For this review, take the finished solid that the model builds, in its own axes (mm). A direction names the side the tool comes from. Round coordinates to 2 decimals unless told otherwise and drop trailing zeros. Write each loop counter-clockwise with the first axis right and the second up, starting at its lowest first coordinate (ties: lowest second). Pieces come first, ordered by that corner, then holes. Notation, with made-up numbers: M 2,42.5 L 42,42.5 A25 ccw 42,72.5 Z; hole C 59,-19 d7. An arc over 180 degrees is marked long. Use one line per item in the form item = value. Start each with the question number.
Item 1: For faces 5 (the cylindrical face through (-0.43, 36.18, 19.26)), 6 (the cylindrical face through (-0.16, -36.18, 22.38)), 7 (the flat face through (0, 39.933, 32)), list the 3-axis set-ups (+Z, -Z, +X, -X, +Y, -Y) from which the entire face can be reached by the end or side of a thin tool; tool diameter is ignored.
Item 2: For line 1 (X direction, y = 9, z = 13.5); line 2 (Y direction, x = 7.5, z = 16); line 3 (Y direction, x = 28, z = 10.5), list the stretches that pass through material, from the lowest coordinate up. Write a range as [from, to].
Item 3: Add section A-A (y = 0). State the section outline as (x, z) points.
Item 4: Draft analysis for pull direction X (two halves, no side actions). For faces 1 (the cylindrical face through (-0.15, -0.559, 33.453)), 2 (the flat face through (51.073, 0, 22)), 3 (the cylindrical face through (-22.66, -4.07, 22.92)), 4 (the flat face through (1, 32.313, 18)), state which applies: released by +X, released by -X, zero draft, split by the parting line, or undercut.
Item 5: Add section C-C (z = 8.5). State the section outline as (x, y) points, and give its area (4 significant figures).
Item 6: Add section B-B (z = 36). State the section outline as (x, y) points.
Item 7: Add section D-D (y = 17). State the section outline as (x, z) points.
Item 8: For P1, Ø4, axis at x = -30, z = 21, coming from the -Y side; P2, Ø10, axis at x = -11, z = 14.5, coming from the +Y side, all flat-tipped, find the tip position at first contact; note any pin that passes through.
from build123d import *

# Parameters (mm, degrees)
F0_W      = 102.14658
F0_H      = 79.865314
F1_DEPTH  = 45.212
F3_DEPTH  = 7.62
F5_DEPTH  = 7.62
F8_DEPTH  = 240.792
F9_R      = 10.614666
F9_R_2    = 10.738577
F10_DEPTH = 83.566


with BuildPart() as f1:
    # F0 (on Top) → F1 (new body)
    with BuildSketch(Plane.XY):
        Rectangle(F0_W, F0_H)
    extrude(amount=F1_DEPTH)

    # F2 (on face) → F3 (cut)
    with BuildSketch(Plane(origin=(0, 39.932657, 0), x_dir=(-1, 0, 0), z_dir=(0, 1, 0))):
        with BuildLine():
            ThreePointArc((30.067937, 45.212), (-0.178194, 19.253555), (-30.424325, 45.212))
            Line((-30.424325, 45.212), (-51.07329, 45.212))
            Line((-51.07329, 45.212), (-51.07329, 0))
            Line((-51.07329, 0), (51.07329, 0))
            Line((51.07329, 0), (51.07329, 45.212))
            Line((51.07329, 45.212), (30.067937, 45.212))
        make_face()
    extrude(amount=-F3_DEPTH, mode=Mode.SUBTRACT)

    # F4 (on face) → F5 (cut)
    with BuildSketch(Plane.XZ.offset(39.932657)):
        with BuildLine():
            ThreePointArc((28.876837, 45.212), (-0.72209, 22.375665), (-30.321017, 45.212))
            Line((-30.321017, 45.212), (-51.07329, 45.212))
            Line((-51.07329, 45.212), (-51.07329, 0))
            Line((-51.07329, 0), (51.07329, 0))
            Line((51.07329, 0), (51.07329, 45.212))
            Line((51.07329, 45.212), (28.876837, 45.212))
        make_face()
    extrude(amount=-F5_DEPTH, mode=Mode.SUBTRACT)

    # F7 (on face) → F8 (cut)
    with BuildSketch(Plane.XZ.offset(39.932657)):
        with BuildLine():
            Line((11.198889, 45.212), (-10.991339, 45.212))
            ThreePointArc((-10.991339, 45.212), (0.103775, 33.44965), (11.198889, 45.212))
        make_face()
    extrude(amount=-F8_DEPTH, mode=Mode.SUBTRACT)

    # F9 (on face) → F10 (cut)
    with BuildSketch(Plane.XY.offset(45.212)):
        with Locations((-32.461744, 0)):
            Circle(F9_R)
        with Locations((31.800803, 0)):
            Circle(F9_R_2)
    extrude(amount=-F10_DEPTH, mode=Mode.SUBTRACT)


solid = f1.part
Calculated:
q1.face_5 = -Z, +Y
q1.face_6 = -Z, -Y
q1.face_7 = +Z, -Z, +X, -X, +Y
q2.line_1 = [-51.07, -38.09], [-26.83, 25.94], [37.66, 51.07]
q2.line_2 = [-32.31, 32.31]
q2.line_3 = [-32.31, -10.04], [10.04, 32.31]
q3.outline = M -51.07,0 L -43.08,0 L -43.08,45.21 L -51.07,45.21 Z; M -21.85,0 L 21.06,0 L 21.06,45.21 L 11.2,45.21 A11.11 cw long -10.99,45.21 L -21.85,45.21 Z; M 42.54,0 L 51.07,0 L 51.07,45.21 L 42.54,45.21 Z
q4.face_1 = undercut
q4.face_2 = released by +X
q4.face_3 = undercut
q4.face_4 = zero draft
q5.outline = M -51.07,-32.31 L 51.07,-32.31 L 51.07,32.31 L -51.07,32.31 Z; hole C -32.46,0 d21.23; hole C 31.8,0 d21.48
q5.area = 5,885 mm^2
q6.outline = M -51.07,-32.31 L -26.18,-32.31 L -26.18,-39.93 L -6.98,-39.93 L -6.98,39.93 L -27.11,39.93 L -27.11,32.31 L -51.07,32.31 Z; M 7.19,-39.93 L 24.74,-39.93 L 24.74,-32.31 L 51.07,-32.31 L 51.07,32.31 L 27.46,32.31 L 27.46,39.93 L 7.19,39.93 Z; hole C -32.46,0 d21.23; hole C 31.8,0 d21.48
q7.outline = M -51.07,0 L 51.07,0 L 51.07,45.21 L 11.2,45.21 A11.11 cw long -10.99,45.21 L -51.07,45.21 Z
q8.P1 = -32.31
q8.P2 = 32.31
